```python
from build123d import *

# Parameters (mm, degrees)
EXTRUDE_THIN1_DEPTH          = 5
EXTRUDE_THIN2_DEPTH          = 2
CUT_EXTRUDE_THIN1_DEPTH      = 1
CUT_EXTRUDE_THIN1_DEPTH_BACK = 3.8
BOSS_EXTRUDE1_DEPTH          = 100
FILLET1_R                    = 1.5
CHAMFER1_SIZE                = 0.6


with BuildPart() as part:
    # Sketch1 → Extrude-Thin1 (new body)
    with BuildSketch(Plane(origin=(0, 0, 0), x_dir=(0, 0, -1), z_dir=(1, 0, 0))):
        Polygon((50, 77), (-50, 77), (-50, 72), (-39, 0), (39, 0), (50, 72), align=None)
        Polygon((46.8, 73.8), (-46.8, 73.8), (-46.8, 72.243034455), (-36.251758625, 3.2), (36.251758625, 3.2), (46.8, 72.243034455), align=None, mode=Mode.SUBTRACT)
    extrude(amount=EXTRUDE_THIN1_DEPTH)

    # Sketch3 → Extrude-Thin2 (add)
    with BuildSketch(Plane(origin=(5, 0, 0), x_dir=(0, 0, -1), z_dir=(1, 0, 0))):
        Polygon((-47.706752564, 72.733323016), (35.345006061, 2.133323016), (37.158511189, 4.266676984), (-45.893247436, 74.866676984), align=None)
        Polygon((45.893247436, 74.866676984), (-37.158511189, 4.266676984), (-35.345006061, 2.133323016), (47.706752564, 72.733323016), align=None)
    extrude(amount=-EXTRUDE_THIN2_DEPTH)

    # Sketch4 → Cut-Extrude-Thin1 (cut, two sides)
    with BuildSketch(Plane.ZY) as cut_extrude_thin1_sk:
        Polygon((50, 77), (50, 72), (39, 0), (-39, 0), (-50, 72), (-50, 77), align=None)
        Polygon((48.8, 75.8), (48.8, 72.091137921), (37.969409484, 1.2), (-37.969409484, 1.2), (-48.8, 72.091137921), (-48.8, 75.8), align=None, mode=Mode.SUBTRACT)
    extrude(amount=CUT_EXTRUDE_THIN1_DEPTH, mode=Mode.SUBTRACT)
    extrude(cut_extrude_thin1_sk.sketch, amount=-CUT_EXTRUDE_THIN1_DEPTH_BACK, mode=Mode.SUBTRACT)

    # Sketch5 → Boss-Extrude1 (add)
    with BuildSketch(Plane(origin=(0, 0, -50), x_dir=(-1, 0, 0), z_dir=(0, 0, -1))):
        with BuildLine():
            Line((-5, 77), (-3.8, 77))
            ThreePointArc((-3.8, 77), (-4.4, 77.6), (-5, 77))
        make_face()
    extrude(amount=-BOSS_EXTRUDE1_DEPTH)

    # Fillet1
    fillet1_edges = [part.edges().sort_by_distance(p)[0] for p in [
        (4, 73.8, -44.638440079),
        (4, 73.8, 44.638440079),
        (4, 71.92064886, -46.750746645),
        (4, 4.826274454, -36.500217222),
        (4, 3.2, 34.090198704),
        (4, 3.2, -34.090198704),
        (4, 4.826274454, 36.500217222),
        (4, 71.92064886, 46.750746645),
    ]]
    fillet(fillet1_edges, radius=FILLET1_R)

    # Chamfer1
    chamfer1_edges = [part.edges().sort_by_distance(p)[0] for p in [
        (5, 37.716457047, 41.525106229),
        (5, 3.2, 0),
        (5, 51.667563114, 22.92561366),
        (5, 73.8, 0),
        (5, 53.505615047, 20.764723924),
        (5, 37.716457047, -41.525106229),
        (5, 51.667563114, -22.92561366),
        (5, 53.505615047, -20.764723924),
        (5, 6.30509587, 35.948092357),
        (5, 4.18245884, 31.417574766),
        (5, 69.485539395, 45.392056481),
        (5, 72.81754116, 41.965816141),
        (5, 69.485539395, -45.392056481),
        (5, 72.81754116, -41.965816141),
        (5, 4.18245884, -31.417574766),
        (5, 6.30509587, -35.948092357),
        (5, 20.292048094, -18.306737062),
        (5, 19.011001017, -15.490603236),
        (5, 20.292048094, 18.306737062),
        (5, 19.011001017, 15.490603236),
    ]]
    chamfer(chamfer1_edges, length=CHAMFER1_SIZE)


solid = part.part
```
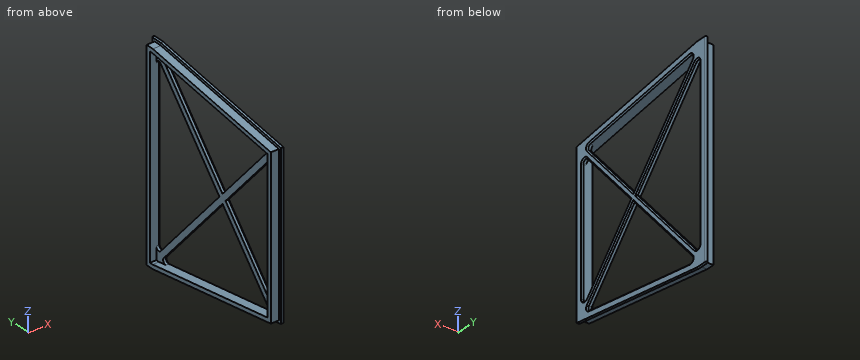
Read the model definition and answer for the solid it produces. Units are mm, in the model's axes. Coordinates: 2 decimals unless noted, no trailing zeros. Loops run counter-clockwise (first coordinate to the right, second up) from the corner with the lowest first, then second, coordinate; pieces in that order, holes last. Notation, with made-up numbers: (52.25, -21) -> (70.25, -21) arc R32 cw to (70.25, 18) -> close; hole circle Ø11 at (66.25, 73.5). An arc over 180 degrees is marked (long way). Return JSON: item names as keys, results as strings.
Item 1: Find section B-B (y = 39). Determine the outline of the cut face in (x, z).
Answers:
{"outline": "(0, -43.74) -> (3.8, -43.74) -> (3.8, -44.96) -> (5, -44.96) -> (5, -42.33) -> (4.4, -41.72) -> (0, -41.72) -> close; (0, 41.72) -> (4.4, 41.72) -> (5, 42.33) -> (5, 44.96) -> (3.8, 44.96) -> (3.8, 43.74) -> (0, 43.74) -> close; (3, -8.02) -> (4.4, -8.02) -> (5, -7.1) -> (5, -4.63) -> (4.4, -3.7) -> (3, -3.7) -> close; (3, 3.7) -> (4.4, 3.7) -> (5, 4.63) -> (5, 7.1) -> (4.4, 8.02) -> (3, 8.02) -> close"}
Item 2: Find the intervals of material crossed by probe 1 along Y at (x, z) = (0.8, 16); probe 2 along Y at (x, z) = (4.3, 2.5); probe 3 along Y at (x, z) = (4.2, 23.5), in increasing order.
Answers:
{"probe 1": "y = 1.2 to 3.2, 73.8 to 75.8", "probe 2": "y = 0 to 3.2, 30.05 to 33.73, 34.3 to 37.98, 73.8 to 77.59", "probe 3": "y = 0 to 3.2, 12.2 to 15.88, 52.16 to 55.83, 73.8 to 77.57"}
Item 3: Flat-ended cylindrical pins translate along their axes: P1, Ø1.1, axis at x = 2.5, z = 10.5, coming from the +Y side; P2, Ø1.9, axis at x = 1, y = 74.5, coming from the -Z side; P3, Ø1.9, axis at x = 1, z = -10.5, coming from the -Y side; P4, Ø12, axis at y = 59.5, z = 15.5, coming from the +X side. Find the tip coordinate at first contact, or state that the pin passes through.
Answers:
{"P1": "stops at y = 75.8", "P2": "stops at z = -48.8", "P3": "stops at y = 1.2", "P4": "passes through"}
Item 4: Find section A-A (x = 1.6). Determine the outline of the cut face in (y, z), plus the area to 3 significant figures.
Answers:
{"outline": "(1.2, -37.97) -> (72.09, -48.8) -> (75.8, -48.8) -> (75.8, 48.8) -> (72.09, 48.8) -> (1.2, 37.97) -> close; hole (3.2, -36.25) -> (72.24, -46.8) -> (73.8, -46.8) -> (73.8, 46.8) -> (72.24, 46.8) -> (3.2, 36.25) -> close", "area": "633 mm2"}
